Part model, mm, in its own coordinate system. Face numbers are marked on the shaded views. A direction names the side the tool comes from. Coordinates: 2 decimals unless noted, no trailing zeros. Order: outer loops, then holes, each group sorted by start corner. A loop starts at its lowest first (then second) coordinate and runs counter-clockwise, first axis right, second up. Notation, with made-up numbers: M -40,74 L -32,74 A9 cw -32,87 Z; hole C -35,-17 d5. An arc over 180 degrees is marked long. Write item = value, one per line. Start each with the question number.
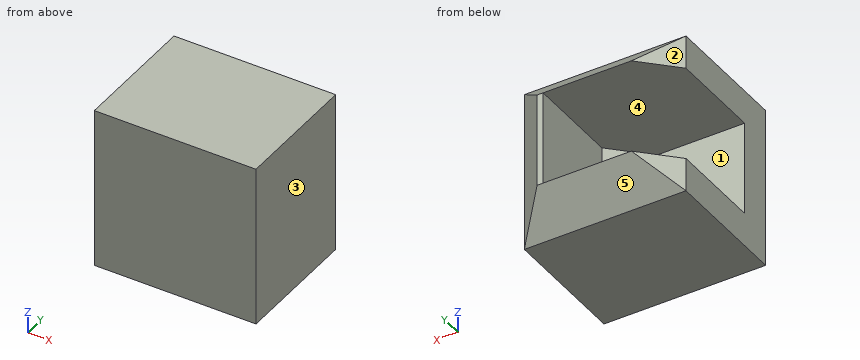
from build123d import *

# Parameters (mm, degrees)
F0_W     = 609.6
F0_H     = 609.6
F1_DEPTH = 609.6
F2_SIZE  = 127
F3_W     = 228.6
F3_H     = 355.6
F3_W_2   = 127
F3_W_3   = 351.28561
F4_DEPTH = 459.74
F5_SIZE  = 127


with BuildPart() as f1:
    # F0 (on Top) → F1 (new body)
    with BuildSketch(Plane.XY):
        with Locations((281.144673, 257.611539)):
            Rectangle(F0_W, F0_H)
    extrude(amount=F1_DEPTH)

    # F2
    f2_edges = [f1.edges().sort_by_distance(p)[0] for p in [
        (585.944673, 562.411539, 304.8),
        (-23.655327, 562.411539, 304.8),
        (281.144673, 562.411539, 0),
        (281.144673, 562.411539, 609.6),
    ]]
    chamfer(f2_edges, length=F2_SIZE)

    # F3 (on face) → F4 (cut)
    with BuildSketch(Plane(origin=(-23.655327, 0, 0), x_dir=(0, -1, 0), z_dir=(-1, 0, 0))):
        with Locations((-194.111539, 304.8)):
            Rectangle(F3_W, F3_H)
        with Locations((-371.911539, 304.8)):
            Rectangle(F3_W_2, F3_H)
        with Locations((-611.054344, 304.8)):
            Rectangle(F3_W_3, F3_H)
    extrude(amount=-F4_DEPTH, mode=Mode.SUBTRACT)

    # F5
    f5_edges = [f1.edges().sort_by_distance(p)[0] for p in [
        (436.084673, 79.811539, 304.8),
    ]]
    chamfer(f5_edges, length=F5_SIZE)


solid = f1.part
Item 1: Cut at C-C, the plane z = 107.5. Write the cut outline in (x, y).
Item 2: Pull direction Z, two halves, no side cores. Call the marked faces 3, 4 and 5: pulls with the +Z half, pulls with the -Z half, needs draft (parallel to the pull), parting line crosses it, or undercut.
Item 3: Cut at B-B, the plane z = 242. Write the cut outline in (x, y), and give its area (3 significant figures).
Item 4: Flat gauge pin, fed straight in: pin 1 (10 mm diameter, centred on x = 347, z = 330, fed in from +Y). Where does the tip first touch, or does it go through?
Item 5: Cut at A-A, the plane x = 250. Write the cut outline in (y, z), and give its area (3 significant figures).
Item 6: Wall check: line 1 along Z through (x, y) = (424.5, 356); line 2 along X through (y, z) = (217, 479); line 3 along Y through (x, z) = (211, 144.5). Give the ranges that are in metal, low to high. Write a range as [from, to].
Item 7: 3-axis set-ups, long thin cutter, end or side, ignore diameter. For the marked faces 1 and 2: which of +Z, -Z, +X, -X, +Y, -Y reach the whole face in a straight line?
Filled sheet:
q1.outline = M -23.66,-47.19 L 585.94,-47.19 L 585.94,435.41 L 478.44,542.91 L 83.84,542.91 L -23.66,435.41 Z
q2.face_3 = needs draft
q2.face_4 = undercut
q2.face_5 = pulls with the -Z half
q3.outline = M -23.66,-47.19 L 585.94,-47.19 L 585.94,435.41 L 458.94,562.41 L 436.08,562.41 L 436.08,206.81 L 309.08,79.81 L -23.66,79.81 Z
q3.area = 150,000 mm2
q4.pin_1 = 122.73
q5.outline = M -47.19,0 L 435.41,0 L 562.41,127 L 79.81,127 L 79.81,482.6 L 562.41,482.6 L 435.41,609.6 L -47.19,609.6 Z
q5.area = 184,000 mm2
q6.line_1 = [0, 127], [482.6, 609.6]
q6.line_2 = [436.08, 585.94]
q6.line_3 = [-47.19, 79.81]
q7.face_1 = -X, +Y
q7.face_2 = +Z, -Z, -X, +Y
